from build123d import *

# Parameters (mm, degrees)
SKETCH059_R     = 3.9
PAD013_DEPTH    = 10
SKETCH060_R     = 7
PAD014_DEPTH    = 8
SKETCH061_R     = 3.5
POCKET033_DEPTH = 6
SKETCH062_R     = 7
SKETCH062_R_2   = 5.1
PAD015_DEPTH    = 10
PAD016_DEPTH    = 3
FILLET014_R     = 2
FILLET015_R     = 1
FILLET016_R     = 1


with BuildPart() as part:
    # Sketch059 → Pad013 (new body)
    with BuildSketch(Plane.XY):
        Circle(SKETCH059_R)
    extrude(amount=PAD013_DEPTH)

    # Sketch060 → Pad014 (join)
    with BuildSketch(Plane.XY.offset(10)):
        Circle(SKETCH060_R)
    extrude(amount=PAD014_DEPTH)

    # Sketch061 → Pocket033 (cut)
    with BuildSketch(Plane.XY.offset(18)):
        Circle(SKETCH061_R)
    extrude(amount=-POCKET033_DEPTH, mode=Mode.SUBTRACT)

    # Sketch062 → Pad015 (join)
    with BuildSketch(Plane.XY.offset(10)):
        Circle(SKETCH062_R)
        Circle(SKETCH062_R_2, mode=Mode.SUBTRACT)
    extrude(amount=-PAD015_DEPTH)

    # Sketch063 → Pad016 (join)
    with BuildSketch(Plane.XY.offset(18)):
        Polygon((6, 2), (7.5, 2), (7.5, 4), (10, 4), (10, 2), (10, -2), (6, -2), align=None)
    extrude(amount=-PAD016_DEPTH)

    # Fillet014
    fillet014_edges = [part.edges().sort_by_distance(p)[0] for p in [
        (10, -2, 16.5),
    ]]
    fillet(fillet014_edges, radius=FILLET014_R)

    # Fillet015
    fillet015_edges = [part.edges().sort_by_distance(p)[0] for p in [
        (6.708204, -2, 16.5),
    ]]
    fillet(fillet015_edges, radius=FILLET015_R)

    # Fillet016
    fillet016_edges = [part.edges().sort_by_distance(p)[0] for p in [
        (7.104102, 2, 15),
        (7.5, 3, 15),
        (7.104102, 2, 18),
        (7.5, 3, 18),
    ]]
    fillet(fillet016_edges, radius=FILLET016_R)


solid = part.part
The model under review builds one solid part; all positions refer to its coordinate system, in mm. A direction names the side the tool comes from. Coordinates: 2 decimals unless noted, no trailing zeros. Write each loop counter-clockwise with the first axis right and the second up, starting at its lowest first coordinate (ties: lowest second). Pieces come first, ordered by that corner, then holes. Notation, with made-up numbers: (64.5, 78) -> (83.5, 78) arc R21 cw to (83.5, 103) -> close; hole circle Ø5 at (86.25, 21). An arc over 180 degrees is marked (long way). Answer in a Markdown table with one row per item.
1. Draft analysis for pull direction Y (two halves, no side actions). For faces 1 (the flat face through (-1, -4, 10)), 2 (the cylindrical face through (6.466, -2.681, 9.126)), 3 (the cylindrical face through (6.86, -2.17, 16.52)), state which applies: +Y half, -Y half, draft (parallel to the pull), parting line (faces both ways), or undercut.
Answers below:
| item | result |
|---|---|
| face 1 | undercut |
| face 2 | parting line |
| face 3 | -Y half |
2. Wall thickness on probe 1 along Y at (x, z) = (0, 16.15); probe 2 along X at (y, z) = (3.5, 3); probe 3 along X at (y, z) = (-2, 7.5): over which ranges is each line inside the solid? List them lowest first. Write a range as [from, to].
Answers below:
| item | result |
|---|---|
| probe 1 | y = [-7, -3.5], [3.5, 7] |
| probe 2 | x = [-6.06, -3.71], [-1.72, 1.72], [3.71, 6.06] |
| probe 3 | x = [-6.71, -4.69], [-3.35, 3.35], [4.69, 6.71] |
3. We need section D-D, the plane z = 6.5. State the section outline as (x, y) points.
Answers below:
| item | result |
|---|---|
| outline | circle Ø14 at (0, 0); circle Ø7.8 at (0, 0); hole circle Ø10.2 at (0, 0) |
4. We need section C-C, the plane x = 0. State the section outline as (y, z) points, and give its area (3 significant figures).
Answers below:
| item | result |
|---|---|
| outline | (-7, 0) -> (-5.1, 0) -> (-5.1, 10) -> (-3.9, 10) -> (-3.9, 0) -> (3.9, 0) -> (3.9, 10) -> (5.1, 10) -> (5.1, 0) -> (7, 0) -> (7, 18) -> (3.5, 18) -> (3.5, 12) -> (-3.5, 12) -> (-3.5, 18) -> (-7, 18) -> close |
| area | 186 mm^2 |
5. We need section B-B, the plane z = 16.5. State the section outline as (x, y) points (3 decimals), and give its area (3 significant figures).
Answers below:
| item | result |
|---|---|
| outline | (6.489, -2.625) arc R1 cw to (7.416, -2) -> (8, -2) arc R2 ccw to (10, 0) -> (10, 4) -> (7.5, 4) -> (7.5, 2) -> (6.708, 2) arc R7 ccw (long way) to start; hole circle Ø7 at (0, 0) |
| area | 132 mm^2 |
6. We need section A-A, the plane y = 3. State the section outline as (x, z) points, and give its area (3 significant figures).
Answers below:
| item | result |
|---|---|
| outline | (-6.32, 0) -> (-4.12, 0) -> (-4.12, 10) -> (-2.49, 10) -> (-2.49, 0) -> (2.49, 0) -> (2.49, 10) -> (4.12, 10) -> (4.12, 0) -> (6.32, 0) -> (6.32, 18) -> (1.8, 18) -> (1.8, 12) -> (-1.8, 12) -> (-1.8, 18) -> (-6.32, 18) -> close; (7.5, 16) arc R1 ccw to (8.5, 15) -> (10, 15) -> (10, 18) -> (8.5, 18) arc R1 ccw to (7.5, 17) -> close |
| area | 180 mm^2 |
7. Clearance check with flat-ended pins moving along their axes: pin 1 Ø1.8 at (x, y) = (7.5, 0.5) entering from -Z; pin 2 Ø2 at (x, z) = (-3.5, 11.5) entering from +Y; pin 3 Ø6 at (x, z) = (7.5, 10.5) entering from -Y; pin 4 Ø1.5 at (y, z) = (5, 11) entering from -X. State where each tip first meets the part, or that it passes through.
Answers below:
| item | result |
|---|---|
| pin 1 | stops at z = 0 |
| pin 2 | stops at y = 6.54 |
| pin 3 | stops at y = -5.36 |
| pin 4 | stops at x = -5.56 |
8. For faces 4 (the flat face through (7.5, 3, 16.5)), 5 (the flat face through (9, 4, 17)), 6 (the cylindrical face through (7.801, 2.854, 17.715)), 7 (the cylindrical face through (7.4, 1.6, 15.2)), list the 3-axis set-ups (+Z, -Z, +X, -X, +Y, -Y) from which the entire face can be reached by the end or side of a thin tool; tool diameter is ignored.
Answers below:
| item | result |
|---|---|
| face 4 | +Z, -Z, +Y |
| face 5 | +Z, -Z, +X, +Y |
| face 6 | +Z, +Y |
| face 7 | -Z, +Y |
